For this review, take the finished solid that the model builds, in its own axes (mm). A direction names the side the tool comes from. Coordinates: 2 decimals unless noted, no trailing zeros. Write each loop counter-clockwise with the first axis right and the second up, starting at its lowest first coordinate (ties: lowest second). Pieces come first, ordered by that corner, then holes. Notation, with made-up numbers: M 20.25,-1 L 61.25,-1 A22 ccw 61.25,26 Z; hole C 50.5,58.25 d8. An arc over 180 degrees is marked long. One line per question, with ' | ' between items.
from build123d import *

# Parameters (mm, degrees)
SKETCH1_W           = 35.56
SKETCH1_H           = 12.7
SKETCH1_R           = 2.38125
BOSS_EXTRUDE1_DEPTH = 3.175
SKETCH7_W           = 35.56
SKETCH7_H           = 3.175
BOSS_EXTRUDE3_DEPTH = 28.575
CUT_EXTRUDE6_DEPTH  = 28.575
FILLET3_R           = 2.54


with BuildPart() as part:
    # Sketch1 → Boss-Extrude1 (new body)
    with BuildSketch(Plane.XY):
        Rectangle(SKETCH1_W, SKETCH1_H)
        with Locations((-12.7, 3.175)):
            Circle(SKETCH1_R, mode=Mode.SUBTRACT)
        with Locations((12.7, 3.175)):
            Circle(SKETCH1_R, mode=Mode.SUBTRACT)
    extrude(amount=BOSS_EXTRUDE1_DEPTH)

    # Sketch7 → Boss-Extrude3 (add)
    with BuildSketch(Plane.XY.offset(3.175)):
        with Locations((0, -4.7625)):
            Rectangle(SKETCH7_W, SKETCH7_H)
    extrude(amount=BOSS_EXTRUDE3_DEPTH)

    # Sketch11 → Cut-Extrude6 (cut)
    with BuildSketch(Plane.XZ.offset(6.35)):
        with BuildLine():
            Line((-6.985, 42.291890454), (6.985, 42.291890454))
            Line((6.985, 42.291890454), (6.985, 21.208109546))
            ThreePointArc((6.985, 21.208109546), (0, 14.223109546), (-6.985, 21.208109546))
            Line((-6.985, 21.208109546), (-6.985, 42.291890454))
        make_face()
        with BuildLine():
            Line((-14.938781825, 28.575), (-9.750668862, 28.575))
            ThreePointArc((-9.750668862, 28.575), (-8.163168862, 26.9875), (-9.750668862, 25.4))
            Line((-9.750668862, 25.4), (-14.938781825, 25.4))
            ThreePointArc((-14.938781825, 25.4), (-16.526281825, 26.9875), (-14.938781825, 28.575))
        make_face()
        with BuildLine():
            Line((14.938781825, 28.575), (9.750668862, 28.575))
            ThreePointArc((9.750668862, 28.575), (8.163168862, 26.9875), (9.750668862, 25.4))
            Line((9.750668862, 25.4), (14.938781825, 25.4))
            ThreePointArc((14.938781825, 25.4), (16.526281825, 26.9875), (14.938781825, 28.575))
        make_face()
    extrude(amount=-CUT_EXTRUDE6_DEPTH, mode=Mode.SUBTRACT)

    # Fillet3
    fillet3_edges = [part.edges().sort_by_distance(p)[0] for p in [
        (6.985, -4.7625, 31.75),
        (17.78, -4.7625, 31.75),
        (-6.985, -4.7625, 31.75),
        (-17.78, -4.7625, 31.75),
        (-17.78, 6.35, 1.5875),
        (17.78, 6.35, 1.5875),
    ]]
    fillet(fillet3_edges, radius=FILLET3_R)


solid = part.part
1) The part is to be moulded in two halves that separate along Z. For faces 5 (the cylindrical face through (14.9, 2.26, 1.57)), 6 (the flat face through (12, -5, 25.4)), 7 (the flat face through (0, 0, 0)), say which applies: +Z half, -Z half, draft (parallel to the pull), parting line (faces both ways), or undercut.
Responses:
face 5: draft | face 6: undercut | face 7: -Z half
2) We need section C-C on z = 19.5. State the section outline as (x, y) points (3 decimals).
Responses:
outline: M -17.78,-6.35 L -6.773,-6.35 L -6.773,-3.175 L -17.78,-3.175 Z; M 6.773,-6.35 L 17.78,-6.35 L 17.78,-3.175 L 6.773,-3.175 Z
3) Insertion check: pin 1 Ø6 at (x, y) = (1.5, -3.5) entering from +Z; pin 2 Ø8.5 at (x, z) = (-6.5, 20.5) entering from +Y (3 decimals); pin 3 Ø3 at (x, y) = (4, -0.5) entering from +Z (3 decimals); pin 4 Ø4 at (x, y) = (12.7, 3.175) entering from +Z. Each pin has a flat end and moves straight along its axis. Give the tip position at first contact, or say it passes through.
Responses:
pin 1: z = 15.87 | pin 2: y = -3.175 | pin 3: z = 3.175 | pin 4: through
4) We need section D-D on x = 14. State the section outline as (y, z) points (3 decimals), then the cut area to 3 significant figures.
Responses:
outline: M -6.35,0 L 1.18,0 L 1.18,3.175 L -3.175,3.175 L -3.175,25.4 L -6.35,25.4 Z; M -6.35,28.575 L -3.175,28.575 L -3.175,31.75 L -6.35,31.75 Z; M 5.17,0 L 6.35,0 L 6.35,3.175 L 5.17,3.175 Z | area: 108 mm^2
5) Machinability: for faces 1 (the flat face through (12, -5, 31.75)), 2 (the flat face through (0, 2, 3.175)), 3 (the flat face through (-6.985, -5, 25)), 4 (the flat face through (-12, -5, 28.575)), which of the approach directions +Z, -Z, +X, -X, +Y, -Y give a long, thin tool a straight path to every point of the face, cutting with its end or side? Answer none if there is none.
Responses:
face 1: +Z, +X, -X, +Y, -Y | face 2: +Z, +X, -X, +Y | face 3: +Z, +Y, -Y | face 4: +Y, -Y
6) To check wall thickness, follow line 1 along X through (y, z) = (3.25, 2.5); line 2 along Z through (x, y) = (-13, -4) (3 decimals); line 3 along X through (y, z) = (-3.5, 26) (3 decimals). State the ranges of each line that lie inside material, in increasing order. Write a range as [from, to].
Responses:
line 1: [-17.78, -15.08], [-10.32, 10.32], [15.08, 17.78] | line 2: [0, 25.4], [28.575, 31.75] | line 3: [-17.78, -16.182], [-8.508, -6.985], [6.985, 8.508], [16.182, 17.78]
7) We need section A-A on x = -12.7. State the section outline as (y, z) points (3 decimals), then the cut area to 3 significant figures.
Responses:
outline: M -6.35,0 L 0.794,0 L 0.794,3.175 L -3.175,3.175 L -3.175,25.4 L -6.35,25.4 Z; M -6.35,28.575 L -3.175,28.575 L -3.175,31.75 L -6.35,31.75 Z; M 5.556,0 L 6.35,0 L 6.35,3.175 L 5.556,3.175 Z | area: 106 mm^2
8) We need section B-B on y = -4.5. State how many separate pieces and enclosed holes the cut face has, then the cut area to 3 significant figures.
Responses:
separate pieces: 1 | enclosed holes: 2 | area: 851 mm^2
